```python
from build123d import *

# Parameters (mm, degrees)
F0_W            = 42
F0_H            = 12
F2_W            = 3.5
F2_H            = 2
F4_R            = 0.3
F6_COPIES_COUNT = 4


# Not quite as in the source:
# - a pattern or mirror of a feature is missing from the dataset's text; its kind, count and spacing are read off the source's solid


with BuildPart() as f1:
    # F0 (on Front) → F1 (revolve)
    with BuildSketch(Plane.XZ):
        with Locations((-21, 7.5)):
            Rectangle(F0_W, F0_H)
    revolve(axis=Axis((-10.2689703926, 0, 0), (1, 0, 0)))

    # F2 (on face) → F3 (revolve, cut)
    with BuildSketch(Plane.XZ):
        with Locations((-16.75, 12.5)):
            Rectangle(F2_W, F2_H)
    revolve(axis=Axis((-21, 0, 0), (-1, 0, 0)), mode=Mode.SUBTRACT)

    # F4
    f4_edges = [f1.edges().sort_by_distance(p)[0] for p in [
        (-18.5, 0, -13.5),
        (-15, 0, -13.5),
        (-18.5, 0, -11.5),
        (-15, 0, -11.5),
    ]]
    fillet(f4_edges, radius=F4_R)

    # F5 (on face) → F6 (revolve, cut)
    with BuildSketch(Plane.XZ):
        Polygon((-15.4035898385, 11.5), (-16.75, 11.5), (-16.75, 0), (-15.75, 0), (-15.75, 11.3), align=None)
    f6 = revolve(axis=Axis((-16.75, 0, 5.75), (0, 0, 1)), mode=Mode.SUBTRACT)

    # F6_copies: F6 ×4 about axis
    f6_copies_axis = Axis((0, 0, 0), (1, 0, 0))
    for i in range(1, F6_COPIES_COUNT):
        add(f6.rotate(f6_copies_axis, i * 360 / F6_COPIES_COUNT), mode=Mode.SUBTRACT)


solid = f1.part
```
Geometry check sheet. Reference: the model listing, model coordinates, mm. A direction names the side the tool comes from. Coordinates: 2 decimals unless noted, no trailing zeros. Order: outer loops, then holes, each group sorted by start corner. A loop starts at its lowest first (then second) coordinate and runs counter-clockwise, first axis right, second up.
Item 1: Mould release check, pull along X, two halves, no side actions. Record for faces 3 (the flat face through (0, 0, -3)), 4 (the cylindrical face through (-30.24, 13.18, -2.93)), 5 (the flat face through (-42, 0, -3)), 6 (the cylindrical face through (-16.73, 3.45, 10.97)): released by +X, released by -X, zero draft, split by the parting line, or undercut.
Item 2: Scan lines: line 1 along Z through (x, y) = (-26, 0); line 2 along X through (y, z) = (0, -7.25). Record each from-to range of solid material in increasing order.
Item 3: Section check C-C (x = -21). Enter the section's corners in (y, z).
Item 4: Depth check by flat-ended pin: pin 1 (2.5 mm diameter, centred on y = 0, z = 0, fed in from -X); pin 2 (8 mm diameter, centred on x = -34.5, z = -8.5, fed in from -Y); pin 3 (1.5 mm diameter, centred on x = -19.5, y = -2.5, fed in from +Z); pin 4 (2 mm diameter, centred on x = -23.5, y = 5.5, fed in from -Z). Enter the tip coordinate at first touch or a pass-through.
Item 5: Section check A-A (x = -16.75). Enter the section's corners in (y, z).
Item 6: Tool access check on faces 1 (the cylindrical face through (-15.796, 0.3, 6.28)), 2 (the flat face through (-15, -7, 10)). Record the directions out of +Z, -Z, +X, -X, +Y, -Y that give a thin tool (end or side, any length) a straight path to the whole face; none if there is none.
Item 7: Section check B-B (y = 0). Count the separate pieces of the cut face and the enclosed holes in it, plus the area to 3 significant figures.
Check sheet entries:
1. face 3: released by +X
1. face 4: zero draft
1. face 5: released by -X
1. face 6: undercut
2. line 1: z = -13.5 to -1.5, 1.5 to 13.5
2. line 2: x = -42 to -17.75, -15.75 to 0
3. outline: circle Ø27 at (0, 0); hole circle Ø3 at (0, 0)
4. pin 1: passes through
4. pin 2: stops at y = -12.73
4. pin 3: stops at z = 13.39
4. pin 4: stops at z = -12.73
5. outline: (-11.43, -1.23) arc R11.5 ccw to (-1.23, -11.43) - (-1, -11.3) - (-1, -1.12) arc R1.5 cw to (-1.12, -1) - (-11.3, -1) - close; (-11.43, 1.23) - (-11.3, 1) - (-1.12, 1) arc R1.5 cw to (-1, 1.12) - (-1, 11.3) - (-1.23, 11.43) arc R11.5 ccw to start; (1, -11.3) - (1.23, -11.43) arc R11.5 ccw to (11.43, -1.23) - (11.3, -1) - (1.12, -1) arc R1.5 cw to (1, -1.12) - close; (1, 1.12) arc R1.5 cw to (1.12, 1) - (11.3, 1) - (11.43, 1.23) arc R11.5 ccw to (1.23, 11.43) - (1, 11.3) - close
6. face 1: +Z, -Z
6. face 2: none
7. separate pieces: 4
7. enclosed holes: 0
7. area: 954 mm2
